Geometry: see drawing. Coordinates: mm, zero at the bounding-box minimum. A direction names the side the tool comes from. Give positions to 0.01 mm unless a question says otherwise; leave off trailing zeros. Loops run counter-clockwise (first coordinate to the right, second up) from the corner with the lowest first, then second, coordinate; pieces in that order, holes last. Notation, with made-up numbers: (-14, 56) -> (20, 56) arc R32 cw to (20, 94) -> close; hole circle Ø2 at (11.25, 7.5). An arc over 180 degrees is marked (long way). One line per question, with ' | ' between items.
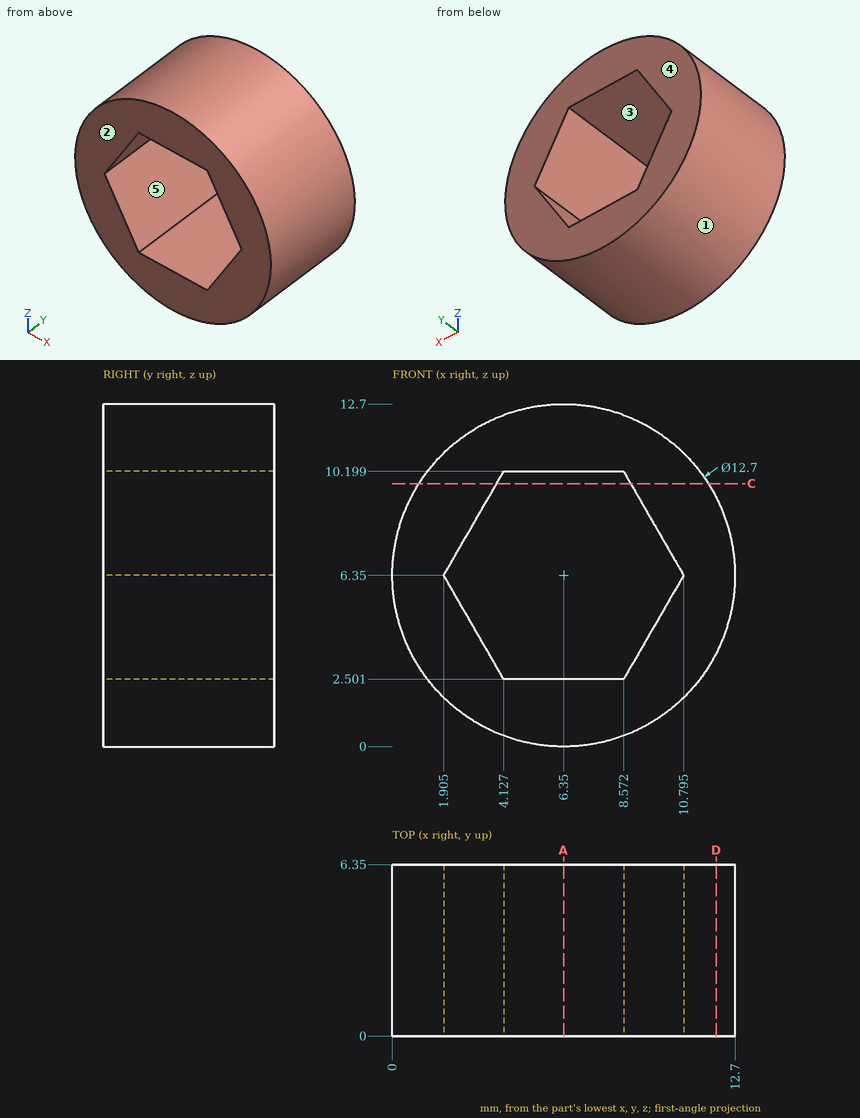
1. Section query C-C (z = 9.75). Output: boundary loops of the cut face in (x, y).
Determined:
outline: (0.99, 0) -> (3.87, 0) -> (3.87, 6.35) -> (0.99, 6.35) -> close; (8.83, 0) -> (11.71, 0) -> (11.71, 6.35) -> (8.83, 6.35) -> close
2. Section query A-A (x = 6.35). Output: boundary loops of the cut face in (y, z).
Determined:
outline: (0, 0) -> (6.35, 0) -> (6.35, 2.5) -> (0, 2.5) -> close; (0, 10.2) -> (6.35, 10.2) -> (6.35, 12.7) -> (0, 12.7) -> close
3. Pull-direction query (Z, two-part tool) for the marked faces 1, 2 and 3; classes: pulls with the +Z half, pulls with the -Z half, needs draft (parallel to the pull), parting line crosses it, or undercut.
Determined:
face 1: parting line crosses it | face 2: needs draft | face 3: undercut
4. Reachability of the marked faces 4 and 5 from +Z, -Z, +X, -X, +Y, -Y: full face, straight path, thin tool, end or side. Return the list, or none.
Determined:
face 4: +Z, -Z, +X, -X, +Y | face 5: +Y, -Y
5. Section query D-D (x = 12). Output: boundary loops of the cut face in (y, z), then the cut area to 3 significant figures.
Determined:
outline: (0, 3.45) -> (6.35, 3.45) -> (6.35, 9.25) -> (0, 9.25) -> close | area: 36.8 mm2
6. Ray query, line 1 along Z through (x, y) = (6.5, 5.75); line 2 along X through (y, z) = (4.5, 5.25) (1 decimal); line 3 along X through (y, z) = (3.25, 3) (1 decimal). Return the intervals inside material, ascending. Write a range as from..to.
Determined:
line 1: z = 0..2.5, 10.2..12.7 | line 2: x = 0.1..2.5, 10.2..12.6 | line 3: x = 1..3.8, 8.9..11.7
7. Pin query (flat end, axial travel): P1, Ø1.5, axis at x = 10.5, y = 4.5, coming from the +Z side; P2, Ø1.5, axis at y = 2, z = 3, coming from the -X side; P3, Ø1.5, axis at x = 8.5, y = 0.5, coming from the +Z side. Return the tip coordinate at first contact, or that it passes through.
Determined:
P1: stops at z = 11.71 | P2: stops at x = 0.56 | P3: stops at z = 12.54
